from build123d import *

# Parameters (mm, degrees)
SKETCH1_R           = 11.24712
BOSS_EXTRUDE2_DEPTH = 5.08


with BuildPart() as part:
    # Sketch1 → Boss-Extrude2 (new body)
    with BuildSketch(Plane.XY):
        with BuildLine():
            Line((-16.134114125, 0), (-8.597805797, 13.053268926))
            ThreePointArc((-8.597805797, 13.053268926), (0, 10.749493806), (8.597805797, 13.053268926))
            Line((8.597805797, 13.053268926), (16.134114125, 0))
            Line((16.134114125, 0), (28.834114125, 0))
            Line((28.834114125, 0), (16.134114125, 21.997045256))
            ThreePointArc((16.134114125, 21.997045256), (0, 45.140716994), (-16.134114125, 21.997045256))
            Line((-16.134114125, 21.997045256), (-28.834114125, 0))
            Line((-28.834114125, 0), (-16.134114125, 0))
        make_face()
        with Locations((0, 27.9451054)):
            Circle(SKETCH1_R, mode=Mode.SUBTRACT)
    extrude(amount=BOSS_EXTRUDE2_DEPTH)


solid = part.part
Input: part model. Units: mm. Frame: model coordinates. A direction names the side the tool comes from. Coordinates: 2 decimals unless noted, no trailing zeros. Loops run counter-clockwise (first coordinate to the right, second up) from the corner with the lowest first, then second, coordinate; pieces in that order, holes last.
Q1. Set-up query: faces 1 (the face through (-12.419, 6.435, 2.504)), 2 (the face through (-7, 18, 0)). Return all of +Z, -Z, +X, -X, +Y, -Y with unobstructed straight access to the full face (end or side cutting, diameter ignored); none if empty.
Q2. Contact query for flat-ended pins moving along their axis: pin 1 (1 mm diameter, centred on y = 31.5, z = 1.5, fed in from +X); pin 2 (3 mm diameter, centred on y = 25, z = 1.5, fed in from +X). Output: stop coordinate, or through.
Q3. Draft query along X for faces 3 (the face through (-22.395, 11.153, 2.504)), 4 (the face through (-23, 0, 3)), 5 (the face through (12.31, 6.62, 2.5)). Return one class per face: +X half, -X half, draft (parallel to the pull), parting line (faces both ways), or undercut.
Q4. Cut plane C-C (z = 0.85). Output: boundary loops of the cut face in (x, y).
Q5. Cut plane A-A (x = 0). Output: boundary loops of the cut face in (y, z), then the cut area to 3 significant figures.
Q6. Cut plane B-B (y = 33). Output: boundary loops of the cut face in (x, z), then the cut area to 3 significant figures.
Q7. Cut plane D-D (x = 15). Output: boundary loops of the cut face in (y, z).
Q8. Material intervals for line 1 (Y direction, x = 0, z = 0.45); line 2 (X direction, y = 28.5, z = 3.15); line 3 (X direction, y = 20.5, z = 2.05), sorted ascending.
Working result:
1. face 1: +Z, -Z, -Y
1. face 2: -Z, +X, -X, +Y, -Y
2. pin 1: stops at x = 16.92
2. pin 2: stops at x = 17.13
3. face 3: -X half
3. face 4: draft
3. face 5: undercut
4. outline: (-28.83, 0) - (-16.13, 0) - (-8.6, 13.05) arc R17.2 ccw to (8.6, 13.05) - (16.13, 0) - (28.83, 0) - (16.13, 22) arc R17.2 ccw (long way) to (-16.13, 22) - close; hole circle Ø22.49 at (0, 27.95)
5. outline: (10.75, 0) - (16.7, 0) - (16.7, 5.08) - (10.75, 5.08) - close; (39.19, 0) - (45.14, 0) - (45.14, 5.08) - (39.19, 5.08) - close
5. area: 60.4 mm2
6. outline: (-16.44, 0) - (-10.05, 0) - (-10.05, 5.08) - (-16.44, 5.08) - close; (10.05, 0) - (16.44, 0) - (16.44, 5.08) - (10.05, 5.08) - close
6. area: 64.9 mm2
7. outline: (1.96, 0) - (36.35, 0) - (36.35, 5.08) - (1.96, 5.08) - close
8. line 1: y = 10.75 to 16.7, 39.19 to 45.14
8. line 2: x = -17.19 to -11.23, 11.23 to 17.19
8. line 3: x = -17 to -8.43, 8.43 to 17
